from build123d import *

# Parameters (mm, degrees)
BASE_SKETCH_W           = 304.8
BASE_SKETCH_H           = 609.6
BOSS_EXTRUDE1_DEPTH     = 11.81
JOINT_X_W               = 25.4
JOINT_X_H               = 11.81
CUT_EXTRUDE1_DEPTH      = 536.943693755
LPATTERN1_COUNT         = 3
LPATTERN1_PITCH         = 139.7
MIRROR1_COPY_1_SKETCH_W = 25.4
MIRROR1_COPY_1_SKETCH_H = 11.81
MIRROR1_COPY_1_DEPTH    = 536.943693755
MIRROR1_COPY_2_SKETCH_W = 25.4
MIRROR1_COPY_2_SKETCH_H = 11.81
MIRROR1_COPY_2_DEPTH    = 536.943693755
JOINT_Y_W               = 11.81
JOINT_Y_H               = 25.4
CUT_EXTRUDE2_DEPTH      = 536.943693755
LPATTERN3_COUNT         = 3
LPATTERN3_PITCH         = 280.29
MIRROR4_COPY_1_SKETCH_W = 11.81
MIRROR4_COPY_1_SKETCH_H = 25.4
MIRROR4_COPY_1_DEPTH    = 536.943693755
MIRROR4_COPY_2_SKETCH_W = 11.81
MIRROR4_COPY_2_SKETCH_H = 25.4
MIRROR4_COPY_2_DEPTH    = 536.943693755


with BuildPart() as part:
    # Base_Sketch → Boss-Extrude1 (new body)
    with BuildSketch(Plane.XY):
        with Locations((127, 152.399963665)):
            Rectangle(BASE_SKETCH_W, BASE_SKETCH_H)
    extrude(amount=BOSS_EXTRUDE1_DEPTH)

    # Joint_X → Cut-Extrude1 (cut, through all)
    with BuildSketch(Plane.XY.offset(11.81)):
        with Locations((-12.7, -146.495036335)):
            Rectangle(JOINT_X_W, JOINT_X_H)
    cut_extrude1 = extrude(amount=-CUT_EXTRUDE1_DEPTH, mode=Mode.SUBTRACT)

    # LPattern1: Cut-Extrude1 ×3
    with Locations(*[(i * LPATTERN1_PITCH, 0, 0) for i in range(1, LPATTERN1_COUNT)]):
        add(cut_extrude1, mode=Mode.SUBTRACT)

    # Mirror1: Cut-Extrude1 across plane
    add(cut_extrude1.mirror(Plane(origin=(0, 152.399963665, 0), x_dir=(0, 0, 1), z_dir=(0, -1, 0))), mode=Mode.SUBTRACT)

    # Mirror1 copy 1 sketch → Mirror1 copy 1 (cut, through all)
    with BuildSketch(Plane(origin=(139.7, 304.79992733, 11.81), x_dir=(1, 0, 0), z_dir=(0, 0, 1))):
        with Locations((-12.7, 146.495036335)):
            Rectangle(MIRROR1_COPY_1_SKETCH_W, MIRROR1_COPY_1_SKETCH_H)
    extrude(amount=-MIRROR1_COPY_1_DEPTH, mode=Mode.SUBTRACT)

    # Mirror1 copy 2 sketch → Mirror1 copy 2 (cut, through all)
    with BuildSketch(Plane(origin=(279.4, 304.79992733, 11.81), x_dir=(1, 0, 0), z_dir=(0, 0, 1))):
        with Locations((-12.7, 146.495036335)):
            Rectangle(MIRROR1_COPY_2_SKETCH_W, MIRROR1_COPY_2_SKETCH_H)
    extrude(amount=-MIRROR1_COPY_2_DEPTH, mode=Mode.SUBTRACT)

    # Joint_Y → Cut-Extrude2 (cut, through all)
    with BuildSketch(Plane.XY.offset(11.81)):
        with Locations((-19.495, -127.890036335)):
            Rectangle(JOINT_Y_W, JOINT_Y_H)
    cut_extrude2 = extrude(amount=-CUT_EXTRUDE2_DEPTH, mode=Mode.SUBTRACT)

    # LPattern3: Cut-Extrude2 ×3
    with Locations(*[(0, i * LPATTERN3_PITCH, 0) for i in range(1, LPATTERN3_COUNT)]):
        add(cut_extrude2, mode=Mode.SUBTRACT)

    # Mirror4: Cut-Extrude2 across plane
    add(cut_extrude2.mirror(Plane.ZY.offset(-127)), mode=Mode.SUBTRACT)

    # Mirror4 copy 1 sketch → Mirror4 copy 1 (cut, through all)
    with BuildSketch(Plane(origin=(254, 280.29, 11.81), x_dir=(-1, 0, 0), z_dir=(0, 0, 1))):
        with Locations((-19.495, 127.890036335)):
            Rectangle(MIRROR4_COPY_1_SKETCH_W, MIRROR4_COPY_1_SKETCH_H)
    extrude(amount=-MIRROR4_COPY_1_DEPTH, mode=Mode.SUBTRACT)

    # Mirror4 copy 2 sketch → Mirror4 copy 2 (cut, through all)
    with BuildSketch(Plane(origin=(254, 560.58, 11.81), x_dir=(-1, 0, 0), z_dir=(0, 0, 1))):
        with Locations((-19.495, 127.890036335)):
            Rectangle(MIRROR4_COPY_2_SKETCH_W, MIRROR4_COPY_2_SKETCH_H)
    extrude(amount=-MIRROR4_COPY_2_DEPTH, mode=Mode.SUBTRACT)


solid = part.part
Part model, mm, in its own coordinate system. A direction names the side the tool comes from. Round coordinates to 2 decimals unless told otherwise and drop trailing zeros. Use CSV: the item, a comma, the result in double quotes.
Item 1: Flat gauge pins, fed straight in: P1, Ø6, axis at y = 449.5, z = 5, coming from the -X side; P2, Ø6, axis at y = 150.5, z = 7.5, coming from the -X side; P3, Ø3.5, axis at y = 451.5, z = 6.5, coming from the +X side. Where does each tip first touch, or does it go through?
Results list:
P1,"stops at x = 0"
P2,"stops at x = -13.59"
P3,"stops at x = 254"
Item 2: Pull direction X, two halves, no side cores. Call faces 5 (the flat face through (114.3, -147, 6)), 6 (the flat face through (254, 451, 6)), 7 (the flat face through (274, 139.7, 6)): pulls with the +X half, pulls with the -X half, needs draft (parallel to the pull), parting line crosses it, or undercut.
Results list:
face 5,"undercut"
face 6,"pulls with the +X half"
face 7,"needs draft"
Item 3: Wall check: L1, parallel to Y at x = -4.5, z = 10.5. Give the ranges that are in metal, low to high.
Results list:
L1,"y = -140.59 to 445.39"
Item 4: Tool access for faces 1 (the flat face through (274, 419.99, 6)), 2 (the flat face through (-7, 445.39, 6)), 3 (the flat face through (-20, -115.19, 6)), 4 (the flat face through (267.59, 153, 6)): list every direction of +Z, -Z, +X, -X, +Y, -Y with a clear straight run to the whole face (end or side of a thin tool).
Results list:
face 1,"+Z, -Z, +X, +Y"
face 2,"+Z, -Z, -X, +Y"
face 3,"+Z, -Z, -X, -Y"
face 4,"+Z, -Z, +X"
